Read the model definition and answer for the solid it produces. Units are mm, in the model's axes. A direction names the side the tool comes from. Coordinates: 2 decimals unless noted, no trailing zeros. Order: outer loops, then holes, each group sorted by start corner. A loop starts at its lowest first (then second) coordinate and runs counter-clockwise, first axis right, second up. Notation, with made-up numbers: M 59,14.25 L 112,14.25 A5 ccw 112,21.25 Z; hole C 60.5,58.5 d5. An arc over 180 degrees is marked long. Use a Markdown table: item, result. Add a question column.
1) Find section B-B on x = 0. Write down the section's boundary in (y, z) (3 decimals), plus the area to 3 significant figures.
2) Find section D-D on y = 52.5. Write down the section's boundary in (x, z) (3 decimals), plus the area to 3 significant figures.
3) Each of these flat-tipped pins is pushed along its axis until it touches: pin 1 Ø8 at (y, z) = (32, -4) entering from -X (3 decimals); pin 2 Ø2 at (y, z) = (56, 0) entering from +X (3 decimals). Where does it stop, or does it pass through?
4) Find section A-A on z = 6.5. Write down the section's boundary in (x, y).
5) Find section C-C on z = 0. Write down the section's boundary in (x, y) (3 decimals).
6) For faces 1 (the face through (-7.555, 128.288, 0.992)), 2 (the face through (-3.3, 0, -3.3)), determine the directions among +Z, -Z, +X, -X, +Y, -Y from which every point of the face is accessible in a straight line to the end or side of a thin tool.
7) Find the intervals of material crossed by probe 1 along Y at (x, z) = (-4.75, 0.5); probe 2 along X at (y, z) = (75.5, 0) (3 decimals); probe 3 along X at (y, z) = (88.5, 2.75), in increasing order. Write a range as [from, to].
8) The mould has two halves that part along Y. Classify faces 3 (the face through (-4.34, 62.61, -0.96)), 4 (the face through (0, -2.54, 0)), 5 (the face through (0, 129.54, 0)): released by +Y, released by -Y, zero draft, split by the parting line, or undercut.
from build123d import *

# Parameters (mm, degrees)
SKETCH1_R           = 4.445
BOSS_EXTRUDE1_DEPTH = 127
SKETCH2_R           = 7.62
BOSS_EXTRUDE2_DEPTH = 2.54
BOSS_EXTRUDE3_START = 2.54
SKETCH3_R           = 7.62
BOSS_EXTRUDE3_DEPTH = 2.54


with BuildPart() as part:
    # Sketch1 → Boss-Extrude1 (new body)
    with BuildSketch(Plane(origin=(0, 0, 0), x_dir=(1, 0, 0), z_dir=(0, 1, 0))):
        with Locations(Location((0, 0, 0), (0, 0, 270))):
            Circle(SKETCH1_R)
    extrude(amount=BOSS_EXTRUDE1_DEPTH)

    # Sketch2 → Boss-Extrude2 (add)
    with BuildSketch(Plane.XZ):
        with Locations(Location((0, 0, 0), (0, 0, 270))):
            Circle(SKETCH2_R)
    extrude(amount=BOSS_EXTRUDE2_DEPTH)

    # Sketch3 → Boss-Extrude3 (add)
    with BuildSketch(Plane(origin=(0, 127, 0), x_dir=(1, 0, 0), z_dir=(0, 1, 0)).offset(BOSS_EXTRUDE3_START)):
        with Locations(Location((0, 0, 0), (0, 0, 90))):
            Circle(SKETCH3_R)
    extrude(amount=-BOSS_EXTRUDE3_DEPTH)


solid = part.part
Check result:
| question | item | result |
|---|---|---|
| 1 | outline | M -2.54,-7.62 L 0,-7.62 L 0,-4.445 L 127,-4.445 L 127,-7.62 L 129.54,-7.62 L 129.54,7.62 L 127,7.62 L 127,4.445 L 0,4.445 L 0,7.62 L -2.54,7.62 Z |
| 1 | area | 1,210 mm2 |
| 2 | outline | C 0,0 d8.89 |
| 2 | area | 62.1 mm2 |
| 3 | pin 1 | stops at x = -4.445 |
| 3 | pin 2 | stops at x = 4.445 |
| 4 | outline | M -3.98,-2.54 L 3.98,-2.54 L 3.98,0 L -3.98,0 Z; M -3.98,127 L 3.98,127 L 3.98,129.54 L -3.98,129.54 Z |
| 5 | outline | M -7.62,-2.54 L 7.62,-2.54 L 7.62,0 L 4.445,0 L 4.445,127 L 7.62,127 L 7.62,129.54 L -7.62,129.54 L -7.62,127 L -4.445,127 L -4.445,0 L -7.62,0 Z |
| 6 | face 1 | +Y, -Y |
| 6 | face 2 | none |
| 7 | probe 1 | y = [-2.54, 0], [127, 129.54] |
| 7 | probe 2 | x = [-4.445, 4.445] |
| 7 | probe 3 | x = [-3.49, 3.49] |
| 8 | face 3 | undercut |
| 8 | face 4 | released by -Y |
| 8 | face 5 | released by +Y |
